For this review, take the finished solid that the model builds, in its own axes (mm). Give positions to 0.01 mm unless a question says otherwise; leave off trailing zeros. Order: outer loops, then holes, each group sorted by start corner. A loop starts at its lowest first (then second) coordinate and runs counter-clockwise, first axis right, second up. Notation, with made-up numbers: (75, -7.5) - (111, -7.5) arc R17 ccw to (111, 1.5) - close; hole circle Ø9 at (71.5, 17). An arc over 180 degrees is marked (long way). Use a Markdown table: item, result. Add a question column.
1) We need section B-B on z = 24.5. Write out the cut boundary in (x, y), then the cut area to 3 significant figures.
2) Wall thickness on L1, parallel to X at y = -2.45, z = -15; L2, parallel to Z at x = -104.5, y = -5.15: over which ranges is each line inside the solid? List them lowest first.
3) Clearance check with flat-ended pins moving along their axes: P1, Ø3, axis at y = -3, z = 33.5, coming from the +X side; P2, Ø1.8, axis at x = 197, y = -4, coming from the +Z side; P3, Ø3, axis at x = 103, y = -4, coming from the +Z side. State where each tip first meets the part, or that it passes through.
4) We need section A-A on x = -14.5. Write out the cut boundary in (y, z).
```python
from build123d import *

# Parameters (mm, degrees)
F0_W     = 20
F0_H     = 6
F1_DEPTH = 6


with BuildPart() as f1:
    # F0 (on Front) → F1 (new body)
    with BuildSketch(Plane.XZ):
        Polygon((-194, -30), (194, -30), (194, -10), (200, -10), (200, 10), (194, 10), (194, 30), (170, 30), (150, 30), (130, 30), (110, 30), (90, 30), (70, 30), (50, 30), (30, 30), (10, 30), (-10, 30), (-30, 30), (-50, 30), (-70, 30), (-90, 30), (-110, 30), (-130, 30), (-150, 30), (-170, 30), (-194, 30), (-194, 10), (-200, 10), (-200, -10), (-194, -10), align=None)
        with Locations((-160, 33)):
            Rectangle(F0_W, F0_H)
        with Locations((-120, 33)):
            Rectangle(F0_W, F0_H)
        with Locations((-80, 33)):
            Rectangle(F0_W, F0_H)
        with Locations((-40, 33)):
            Rectangle(F0_W, F0_H)
        with Locations((0, 33)):
            Rectangle(F0_W, F0_H)
        with Locations((40, 33)):
            Rectangle(F0_W, F0_H)
        with Locations((80, 33)):
            Rectangle(F0_W, F0_H)
        with Locations((120, 33)):
            Rectangle(F0_W, F0_H)
        with Locations((160, 33)):
            Rectangle(F0_W, F0_H)
    extrude(amount=F1_DEPTH)


solid = f1.part
```
Checked values:
| question | item | result |
|---|---|---|
| 1 | outline | (-194, -6) - (194, -6) - (194, 0) - (-194, 0) - close |
| 1 | area | 2,330 mm² |
| 2 | L1 | -194 to 194 |
| 2 | L2 | -30 to 30 |
| 3 | P1 | x = 170 |
| 3 | P2 | z = 10 |
| 3 | P3 | z = 30 |
| 4 | outline | (-6, -30) - (0, -30) - (0, 30) - (-6, 30) - close |
